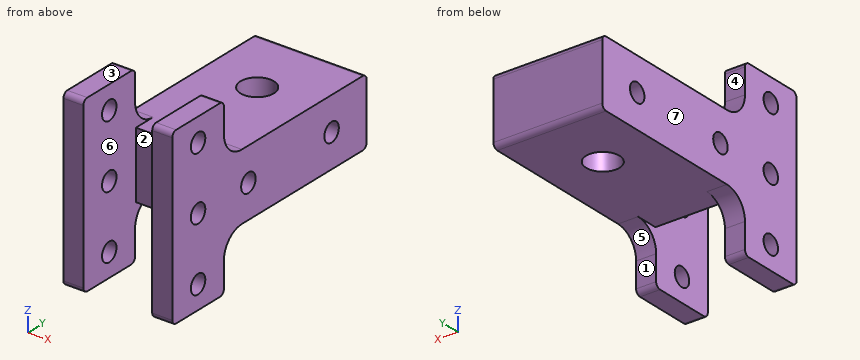
```python
from build123d import *

# Parameters (mm, degrees)
EXTRUDE1_DEPTH      = 10.3
EXTRUDE1_DEPTH_BACK = 10.3
SKETCH1_W           = 20
SKETCH1_H           = 55
EXTRUDE2_DEPTH      = 6
SKETCH4_R           = 2.8
EXTRUDE3_DEPTH      = 78.478061411
SKETCH5_R           = 5
EXTRUDE4_DEPTH      = 77.326797391
FILLET2_R           = 1.5


with BuildPart() as part:
    # Sketch1 → Extrude1 (new, two sides: drawn at the far end of the back side and taken through both)
    with BuildSketch(Plane(origin=(0, 0, 0), x_dir=(0, 0, -1), z_dir=(1, 0, 0)).offset(-EXTRUDE1_DEPTH_BACK)):
        with Locations((0, 37.8)):
            Rectangle(SKETCH1_W, SKETCH1_H)
    extrude(amount=EXTRUDE1_DEPTH + EXTRUDE1_DEPTH_BACK)

    # Sketch2 → Extrude2 (add)
    with BuildSketch(Plane(origin=(10.3, 0, 0), x_dir=(0, 0, -1), z_dir=(1, 0, 0))):
        with BuildLine():
            Line((26, 10), (17, 10))
            ThreePointArc((17, 10), (12.050252532, 12.050252532), (10, 17))
            Line((10, 17), (10, 65.3))
            Line((10, 65.3), (-10, 65.3))
            Line((-10, 65.3), (-10, 17))
            ThreePointArc((-10, 17), (-12.050252532, 12.050252532), (-17, 10))
            Line((-17, 10), (-26, 10))
            Line((-26, 10), (-26, -10))
            Line((-26, -10), (26, -10))
            Line((26, -10), (26, 10))
        make_face()
    extrude2 = extrude(amount=EXTRUDE2_DEPTH)

    # Mirror2: Extrude2 across plane
    add(extrude2.mirror(Plane(origin=(0, 0, 0), x_dir=(0, 0, 1), z_dir=(1, 0, 0))))

    # Sketch4 → Extrude3 (cut, through all)
    with BuildSketch(Plane(origin=(16.3, 0, 0), x_dir=(0, 0, -1), z_dir=(1, 0, 0))):
        Circle(SKETCH4_R)
        with Locations((19, 0)):
            Circle(SKETCH4_R)
        with Locations((-19, 0)):
            Circle(SKETCH4_R)
        with Locations((0, 19.5)):
            Circle(SKETCH4_R)
        with Locations((0, 51.75)):
            Circle(SKETCH4_R)
    extrude(amount=-EXTRUDE3_DEPTH, mode=Mode.SUBTRACT)

    # Sketch5 → Extrude4 (cut, through all)
    with BuildSketch(Plane.XY.offset(10)):
        with Locations((0, 44)):
            Circle(SKETCH5_R)
    extrude(amount=-EXTRUDE4_DEPTH, mode=Mode.SUBTRACT)

    # Fillet2
    fillet2_edges = [part.edges().sort_by_distance(p)[0] for p in [
        (13.3, 10, 26),
        (13.3, -10, 26),
        (13.3, -10, -26),
        (13.3, 10, -26),
        (-13.3, -10, 26),
        (-13.3, 10, 26),
        (-13.3, 10, -26),
        (-13.3, -10, -26),
        (0, 65.3, 10),
        (0, 65.3, -10),
    ]]
    fillet(fillet2_edges, radius=FILLET2_R)


solid = part.part
```
The listing builds one solid part. Answer for the finished solid, in the listing's coordinates (mm). Face numbers are marked on the shaded views. A direction names the side the tool comes from. Coordinates: 2 decimals unless noted, no trailing zeros. Order: outer loops, then holes, each group sorted by start corner. A loop starts at its lowest first (then second) coordinate and runs counter-clockwise, first axis right, second up. Notation, with made-up numbers: M -1.75,26.5 L 18.25,26.5 A27 cw 18.25,44.5 Z; hole C 54.25,-34.5 d2. An arc over 180 degrees is marked long. Answer as a JSON object with one key per item and string values. Group by question number.
1. Section A-A on x = 4 is taken. Write down the section's boundary in (y, z), then the cut area to 3 significant figures.
2. Straight lines are drawn through the part: line 1 (X direction, y = 9.5, z = 22); line 2 (Y direction, x = 13.5, z = -19); line 3 (Y direction, x = 10, z = -0.5) (3 decimals). For each, find the intervals that lie inside material, in ascending order.
3. A tool of negligible diameter and unlimited length cuts with its end or side. For the marked faces 1, 2, 3 and 4, from which of +Z, -Z, +X, -X, +Y, -Y can it reach the whole face along a straight path? Write none if from no direction.
4. Flat-ended cylindrical pins translate along their axes: P1, Ø12, axis at x = 10, y = 46, coming from the +Z side; P2, Ø6, axis at x = 0, y = 44, coming from the -Z side; P3, Ø1.8, axis at x = 12.5, z = -22.5, coming from the +Y side; P4, Ø1, axis at x = 9.5, y = 39, coming from the -Z side. Find the tip coordinate at first contact, or state that the pin passes through.
5. Section D-D on x = 0 is taken. Write down the section's boundary in (y, z).
6. Section C-C on z = 23 is taken. Write down the section's boundary in (x, y), then the cut area to 3 significant figures.
7. Determine the mould class of the marked faces 5, 6 and 7 for opening direction X: released by +X, released by -X, zero draft, split by the parting line, or undercut.
8. Section B-B on y = 19.5 is taken. Write down the section's boundary in (x, z).
Values follow:
{
 "1": {"outline": "M 10.3,-10 L 41,-10 L 41,10 L 10.3,10 Z; M 47,-10 L 63.8,-10 A1.5 ccw 65.3,-8.5 L 65.3,8.5 A1.5 ccw 63.8,10 L 47,10 Z; hole C 19.5,0 d5.6; hole C 51.75,0 d5.6", "area": "930 mm2"},
 "2": {"line 1": "-16.3 to -10.3, 10.3 to 16.3", "line 2": "-10 to -2.8, 2.8 to 10", "line 3": "10.3 to 16.745, 22.255 to 48.995, 54.505 to 65.3"},
 "3": {"face 1": "-Z, +X, -X, +Y", "face 2": "+Z, -Z, -Y", "face 3": "+Z, +X, -X, +Y, -Y", "face 4": "+Z, +X, -X, +Y"},
 "4": {"P1": "z = 10", "P2": "through", "P3": "y = 10", "P4": "z = -10"},
 "5": {"outline": "M 10.3,-10 L 39,-10 L 39,10 L 10.3,10 Z; M 49,-10 L 63.8,-10 A1.5 ccw 65.3,-8.5 L 65.3,8.5 A1.5 ccw 63.8,10 L 49,10 L 49,0.53 A2.8 cw long 49,-0.53 Z; hole C 19.5,0 d5.6"},
 "6": {"outline": "M -16.3,-10 L -10.3,-10 L -10.3,10 L -16.3,10 Z; M 10.3,-10 L 16.3,-10 L 16.3,10 L 10.3,10 Z", "area": "240 mm2"},
 "7": {"face 5": "zero draft", "face 6": "undercut", "face 7": "released by -X"},
 "8": {"outline": "M -16.3,-10 L 16.3,-10 L 16.3,-2.8 L -16.3,-2.8 Z; M -16.3,2.8 L 16.3,2.8 L 16.3,10 L -16.3,10 Z"}
}
